Design review of the part built by this model. Coordinates are the model's own, in mm. A direction names the side the tool comes from. Round coordinates to 2 decimals unless told otherwise and drop trailing zeros. Order: outer loops, then holes, each group sorted by start corner. A loop starts at its lowest first (then second) coordinate and runs counter-clockwise, first axis right, second up. Notation, with made-up numbers: M 57.25,87.5 L 97.25,87.5 A18 ccw 97.25,106.5 Z; hole C 2.25,87 d8. An arc over 180 degrees is marked long. Use a Markdown table: item, result. Add a question column.
(1) Take a section at C-C (y = 8). Write out the cut boundary in (x, z).
(2) Take a section at D-D (z = 13.4). Write out the cut boundary in (x, y).
(3) Machinability: for faces 4 (the face through (-3, 9, 12.691)), 5 (the face through (3.303, 9, 14)), which of the approach directions +Z, -Z, +X, -X, +Y, -Y give a long, thin tool a straight path to every point of the face, cutting with its end or side? Answer none if there is none.
(4) For pin 1 (2 mm diameter, centred on x = -3, y = 8.5, fed in from +Z), flat-tipped, find the tip position at first contact; note if it passes through.
(5) To check wall thickness, follow probe 1 along X at (y, z) = (13, 14); probe 2 along Y at (x, z) = (-7.9, 13.5); probe 3 along X at (y, z) = (9.75, 16.3). State the ranges of each line that lie inside material, in increasing order. Write a range as from..to.
(6) The part is to be moulded in two halves that separate along X. For faces 1 (the face through (-8.372, 9, 14)), 2 (the face through (-7.372, 9, 15)), 3 (the face through (-2, 9, 12.191)), say which applies: released by +X, released by -X, zero draft, split by the parting line, or undercut.
(7) Take a section at A-A (z = 15.6). Write out the cut boundary in (x, y).
(8) Take a section at B-B (x = -1.5). Write out the cut boundary in (y, z).
```python
from build123d import *

# Parameters (mm, degrees)
BOSS_EXTRUDE1_DEPTH = 18
SKETCH5_R           = 0.3
CUT_EXTRUDE1_DEPTH  = 1.5
SKETCH6_R           = 0.3
CUT_EXTRUDE2_DEPTH  = 12.675000001


with BuildPart() as part:
    # Sketch1 → Boss-Extrude1 (new body)
    with BuildSketch(Plane(origin=(0, 0, 0), x_dir=(1, 0, 0), z_dir=(0, 1, 0))):
        Polygon((-8.372296156, -12.19086985), (-8.372296156, -16.69086985), (-8.022296156, -16.69086985), (-8.022296156, -17.44086985), (-7.722296156, -17.44086985), (-7.722296156, -16.69086985), (-7.372296156, -16.69086985), (-7.372296156, -12.69086985), (2.302703845, -12.69086985), (2.302703845, -16.19086985), (2.652703845, -16.19086985), (2.652703845, -16.94086985), (2.952703845, -16.94086985), (2.952703845, -16.19086985), (3.302703845, -16.19086985), (3.302703845, -12.19086985), align=None)
    extrude(amount=BOSS_EXTRUDE1_DEPTH)

    # Sketch5 → Cut-Extrude1 (cut, through all)
    with BuildSketch(Plane.XY.offset(12.69086985)):
        with Locations((-6, 0.6)):
            Circle(SKETCH5_R)
        with Locations((-4.5, 0.6)):
            Circle(SKETCH5_R)
        with Locations((-3, 0.6)):
            Circle(SKETCH5_R)
        with Locations((-1.5, 0.6)):
            Circle(SKETCH5_R)
        with Locations((1.5, 0.6)):
            Circle(SKETCH5_R)
        with Locations((0, 0.6)):
            Circle(SKETCH5_R)
    extrude(amount=-CUT_EXTRUDE1_DEPTH, mode=Mode.SUBTRACT)

    # Sketch6 → Cut-Extrude2 (cut, through all)
    with BuildSketch(Plane(origin=(3.302703845, 0, 0), x_dir=(0, 0, -1), z_dir=(1, 0, 0))):
        with Locations((-15, 0.6)):
            Circle(SKETCH6_R)
        with Locations((-13.5, 0.6)):
            Circle(SKETCH6_R)
    extrude(amount=-CUT_EXTRUDE2_DEPTH, mode=Mode.SUBTRACT)


solid = part.part
```
Verdict:
| question | item | result |
|---|---|---|
| 1 | outline | M -8.37,12.19 L 3.3,12.19 L 3.3,16.19 L 2.95,16.19 L 2.95,16.94 L 2.65,16.94 L 2.65,16.19 L 2.3,16.19 L 2.3,12.69 L -7.37,12.69 L -7.37,16.69 L -7.72,16.69 L -7.72,17.44 L -8.02,17.44 L -8.02,16.69 L -8.37,16.69 Z |
| 2 | outline | M -8.37,0 L -7.37,0 L -7.37,0.32 L -8.37,0.32 Z; M -8.37,0.88 L -7.37,0.88 L -7.37,18 L -8.37,18 Z; M 2.3,0 L 3.3,0 L 3.3,0.32 L 2.3,0.32 Z; M 2.3,0.88 L 3.3,0.88 L 3.3,18 L 2.3,18 Z |
| 3 | face 4 | +Z, +Y, -Y |
| 3 | face 5 | +Z, -Z, +X, +Y, -Y |
| 4 | pin 1 | stops at z = 12.69 |
| 5 | probe 1 | x = -8.37..-7.37, 2.3..3.3 |
| 5 | probe 2 | y = 0..0.3, 0.9..18 |
| 5 | probe 3 | x = -8.37..-7.37, 2.65..2.95 |
| 6 | face 1 | released by -X |
| 6 | face 2 | undercut |
| 6 | face 3 | zero draft |
| 7 | outline | M -8.37,0 L -7.37,0 L -7.37,18 L -8.37,18 Z; M 2.3,0 L 3.3,0 L 3.3,18 L 2.3,18 Z |
| 8 | outline | M 0,12.19 L 0.3,12.19 L 0.3,12.69 L 0,12.69 Z; M 0.9,12.19 L 18,12.19 L 18,12.69 L 0.9,12.69 Z |
